Could you check a few things on this model? Use its own coordinates, in mm. Give positions to 0.01 mm unless a question says otherwise; leave off trailing zeros. Loops run counter-clockwise (first coordinate to the right, second up) from the corner with the lowest first, then second, coordinate; pieces in that order, holes last. Notation, with made-up numbers: (57, 71.5) -> (83, 71.5) arc R8 ccw to (83, 86.5) -> close; hole circle Ø11 at (-1, -16.5). An arc over 180 degrees is marked (long way). Write item = value, one per line. Start each with the question number.
1) I want a section at B-B (z = 0.95). List the corners of the cut face in (x, y) for me.
2) I need wall thicknesses on probe 1 along Y at (x, z) = (7.95, 2.9); probe 2 along X at (y, z) = (-1, 0.35); probe 3 along X at (y, z) = (-2.5, 1.65). Which ranges of each line are inside material? Lowest first, please. Write a range as from..to.
3) I'm going to push flat-ended pins straight in: pin 1 Ø3 at (y, z) = (2, 0.5) entering from +X; pin 2 Ø2.5 at (x, y) = (-7.95, 0) entering from +Z; pin 3 Ø1.7 at (x, y) = (0, 1) entering from +Z; pin 4 Ø1 at (x, z) = (1, -0.5) entering from -Y. Where does each tip first touch, or does it pass through?
4) I want a section at D-D (x = 7.25). List the corners of the cut face in (y, z) for me.
5) If we mould it in two halves opening along X, with no side actions, what happens to faces 1 (the face through (8, 2, 3.5)), 2 (the face through (0, 0, 1.5))? For each: +X half, -X half, draft (parallel to the pull), parting line (faces both ways), or undercut.
6) I want a section at A-A (y = 0). List the corners of the cut face in (x, z) for me.
7) I want a section at C-C (z = 2.45). List the corners of the cut face in (x, y) for me, and give its area (3 significant figures).
from build123d import *
from build123d.topology import SkipClean

# Parameters (mm, degrees)
SKETCH1_R           = 1.5
BOSS_EXTRUDE1_DEPTH = 1.5
SKETCH2_OUTSIDE_W   = 28.48
SKETCH2_OUTSIDE_H   = 12.58
CUT_EXTRUDE1_DEPTH  = 3
BOSS_EXTRUDE2_START = 2
SKETCH3_R           = 3
SKETCH3_R_2         = 1.5
BOSS_EXTRUDE2_DEPTH = 2


with BuildPart() as part:
    # Sketch1 → Boss-Extrude1 (new, symmetric)
    with BuildSketch(Plane.XY):
        with BuildLine():
            Line((-7.95, 3), (7.95, 3))
            ThreePointArc((7.95, 3), (10.95, 0), (7.95, -3))
            Line((7.95, -3), (-7.95, -3))
            ThreePointArc((-7.95, -3), (-10.95, 0), (-7.95, 3))
        make_face()
        with Locations((-7.95, 0)):
            Circle(SKETCH1_R, mode=Mode.SUBTRACT)
        with Locations((7.95, 0)):
            Circle(SKETCH1_R, mode=Mode.SUBTRACT)
    extrude(amount=BOSS_EXTRUDE1_DEPTH, both=True)

    # Sketch2 outside → Cut-Extrude1 (cut)
    with SkipClean():  # the faces are left unmerged after this step: merging them gives an invalid solid
        with BuildSketch(Plane.XY.offset(1.5)):
            Rectangle(SKETCH2_OUTSIDE_W, SKETCH2_OUTSIDE_H)
            with BuildLine():
                ThreePointArc((-6.95625, 2.830629071), (-10.95, 0), (-6.95625, -2.830629071))
                ThreePointArc((-6.95625, -2.830629071), (0, -1.645032568), (6.95625, -2.830629071))
                ThreePointArc((6.95625, -2.830629071), (10.95, 0), (6.95625, 2.830629071))
                ThreePointArc((6.95625, 2.830629071), (0, 1.645032568), (-6.95625, 2.830629071))
            make_face(mode=Mode.SUBTRACT)
        extrude(amount=-CUT_EXTRUDE1_DEPTH, mode=Mode.SUBTRACT)

    # Sketch3 → Boss-Extrude2 (add)
    # profile 1 of 2: a face of its own
    with SkipClean():  # the faces are left unmerged after this step: merging them gives an invalid solid
        with BuildSketch(Plane.XY.offset(1.5).offset(BOSS_EXTRUDE2_START)):
            with Locations(Location((-7.95, 0, 0), (0, 0, 289.344662967))):
                Circle(SKETCH3_R)
            with Locations((-7.95, 0)):
                Circle(SKETCH3_R_2, mode=Mode.SUBTRACT)
        # profile 2 of 2: a face of its own
        with BuildSketch(Plane.XY.offset(1.5).offset(BOSS_EXTRUDE2_START)):
            with Locations(Location((7.95, 0, 0), (0, 0, 250.655337033))):
                Circle(SKETCH3_R)
            with Locations((7.95, 0)):
                Circle(SKETCH3_R_2, mode=Mode.SUBTRACT)
        extrude(amount=-BOSS_EXTRUDE2_DEPTH)


solid = part.part
Answer list:
q1.outline = (-6.96, -2.83) arc R21 cw to (6.96, -2.83) arc R3 ccw (long way) to (6.96, 2.83) arc R21 cw to (-6.96, 2.83) arc R3 ccw (long way) to start; hole circle Ø3 at (-7.95, 0); hole circle Ø3 at (7.95, 0)
q2.probe_1 = -3..-1.5, 1.5..3
q2.probe_2 = -10.78..-9.07, -6.83..6.83, 9.07..10.78
q2.probe_3 = -9.61..-6.29, 6.29..9.61
q3.pin_1 = 10.91
q3.pin_2 = through
q3.pin_3 = 1.5
q3.pin_4 = -1.7
q4.outline = (-2.92, -1.5) -> (-1.33, -1.5) -> (-1.33, 3.5) -> (-2.92, 3.5) -> close; (1.33, -1.5) -> (2.92, -1.5) -> (2.92, 3.5) -> (1.33, 3.5) -> close
q5.face_1 = draft
q5.face_2 = undercut
q6.outline = (-10.95, -1.5) -> (-9.45, -1.5) -> (-9.45, 3.5) -> (-10.95, 3.5) -> close; (-6.45, -1.5) -> (6.45, -1.5) -> (6.45, 3.5) -> (4.95, 3.5) -> (4.95, 1.5) -> (-4.95, 1.5) -> (-4.95, 3.5) -> (-6.45, 3.5) -> close; (9.45, -1.5) -> (10.95, -1.5) -> (10.95, 3.5) -> (9.45, 3.5) -> close
q7.outline = circle Ø6 at (-7.95, 0); circle Ø6 at (7.95, 0); hole circle Ø3 at (-7.95, 0); hole circle Ø3 at (7.95, 0)
q7.area = 42.4 mm^2
